The listing builds one solid part. Answer for the finished solid, in the listing's coordinates (mm). Face numbers are marked on the shaded views. Give positions to 0.01 mm unless a question says otherwise; leave off trailing zeros. Loops run counter-clockwise (first coordinate to the right, second up) from the corner with the lowest first, then second, coordinate; pieces in that order, holes last. Notation, with made-up numbers: (0, 18) - (10, 18) arc R20 cw to (10, 37) - close; hole circle Ø8 at (8.25, 32.5). An arc over 180 degrees is marked (long way). Write each question's results on one line, items separated by ' | '.
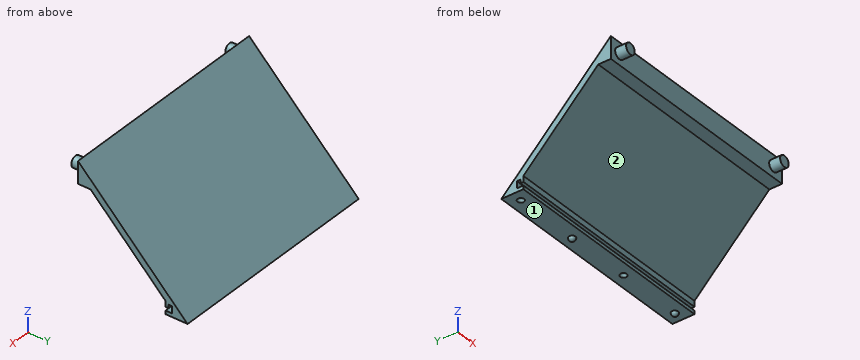
Autodesk Inventor part; units mm, degrees
sketch "Sketch1" plane through (0, 0, 0) normal (1, 0, 0) x (0, 1, 0)
  line L0 (25, 25) -> (-25, 25)
  line L1 (-25, 25) -> (-25, -25)
  line L2 (-25, -25) -> (25, -25)
  line L3 (25, -25) -> (25, 25)
  line L4 (-35, 0) -> (35, 0)
  line L5 (0, 35) -> (0, -35)
  line L6 (-25, 25) -> (25, -25)
  line L7 (-19.2426, 15) -> (14.9373, -19.1799)
  line L8 (-19.2426, 15) -> (-25, 15)
  line L9 (14.9373, -25) -> (14.9373, -19.1799)
  line L10 (14.9373, -21.8) -> (17.9373, -21.8)
  line L11 (17.9373, -21.8) -> (17.9373, -23.4)
  line L12 (17.9373, -23.4) -> (14.9373, -23.4)
  line L13 (14.9373, -23.4) -> (14.9373, -21.8)
  line L14 (17.9373, -21.8) -> (16.3373, -21.8)
  line L15 (16.3373, -21.8) -> (16.3373, -20.2)
  line L16 (16.3373, -20.2) -> (17.9373, -20.2)
  line L17 (17.9373, -20.2) -> (17.9373, -21.8)
  point P0 (0, 0)
  point P1 (25, 0)
  point P2 (0, 25)
  point P3 (20.7574, -25)
  point P4 (-25, 20.7574)
  point P5 (0, 0)
  point P6 (0, 0)
  point P7 (0, -4.2426)
  point P8 (-4.2426, 0)
  dimension "d0" = 50
  dimension "d1" = 50
  dimension "d2" = 3
  dimension "d5" = 10
  dimension "d92" = 3
  dimension "d93" = 1.6
  dimension "d94" = 1.6
  dimension "d95" = 1.6
  dimension "d96" = 1.6
  dimension "d97" = 1.6
extrude "Extrusion1" add sketch "Sketch1" along normal mid plane 100 contours L6 L4 L7 L8 L1 | L5 L7 L4 | L6 L2 L9 L12 L11 L17 L16 L15 L10 L7 L5
sketch "Sketch4" plane through (50, 25, -25) normal (0, 0, -1) x (-1, 0, 0)
  circle A0 centre (5, -5) radius 1.5
  line L0 (0, -10.0627) -> (0, 0)
  line L1 (0, 0) -> (100, 0)
  line L2 (5, -3.5) -> (5, -6.5)
  circle A1 centre (35, -5) radius 1.5
  line L3 (35, -3.5) -> (35, -6.5)
  circle A2 centre (65, -5) radius 1.5
  line L4 (65, -3.5) -> (65, -6.5)
  circle A3 centre (95, -5) radius 1.5
  line L5 (95, -3.5) -> (95, -6.5)
  point P0 (50, -25)
  point P1 (0, -50)
  dimension "d45" = 3
  dimension "d46" = 5
  dimension "d47" = 5
  dimension "d48" = 3
  dimension "d98" = 3
  dimension "d99" = 5
  dimension "d100" = 30
  dimension "d101" = 3
  dimension "d104" = 60
revolve "Revolution2" add sketch "Sketch4" angle 360 about axis through (45, 21.5, -25) along (0, -1, 0) picked at (4.5036, -4.9397) contours L2 A0
revolve "Revolution3" cut sketch "Sketch4" angle 360 about axis through (15, 21.5, -25) along (0, -1, 0) picked at (34.5036, -5.0603) contours L3 A1
revolve "Revolution4" add sketch "Sketch4" angle 360 about axis through (-15, 21.5, -25) along (0, -1, 0) picked at (64.2365, -5.2413) contours L4 A2
revolve "Revolution5" cut sketch "Sketch4" angle 360 about axis through (-45, 21.5, -25) along (0, -1, 0) picked at (94.1238, -4.716) contours L5 A3
sketch "Sketch5" plane through (-50, -25, 15) normal (0, -1, 0) x (1, 0, 0)
  circle A0 centre (5, 5) radius 2.5
  line L0 (0, 0) -> (0, 10)
  line L1 (0, 10) -> (100, 10)
  line L2 (50, 20) -> (50, -50)
  circle A1 centre (95, 5) radius 2.5
  line L3 (0, 5) -> (100, 5)
  line L4 (100, -40) -> (100, 10)
  point P0 (50, -15)
  dimension "d73" = 5
  dimension "d74" = 5
extrude "Extrusion3" add sketch "Sketch5" along normal blind 5 contours L3 A0 | A0 L3 | L3 A1 | A1 L3
properties part number "Roof_Small"
Item 1: Flat-ended cylindrical pins translate along their axes: P1, Ø0.8, axis at x = 24.5, y = 17.5, coming from the -Z side; P2, Ø2.5, axis at x = 12, z = -21, coming from the -Y side; P3, Ø2, axis at x = 29, z = -0.5, coming from the +Y side; P4, Ø12, axis at y = -19, z = -1, coming from the +X side. Find the tip coordinate at first contact, or state that the pin passes through.
Values found:
P1: stops at z = -25 | P2: stops at y = 14.94 | P3: stops at y = 1.5 | P4: passes through
Item 2: Find the intervals of material crossed by line 1 along Z through (x, y) = (-32.5, 16.5); line 2 along Z through (x, y) = (-42, -18); line 3 along Z through (x, y) = (38.5, 17), in increasing order. Write a range as [from, to].
Values found:
line 1: z = [-25, -23.4], [-20.2, -16.5] | line 2: z = [13.76, 18] | line 3: z = [-25, -23.4], [-20.2, -17]
Item 3: A cutting plane is placed at A-A, the plane x = 45. Determine the outline of the cut face in (y, z), plus the area to 3 significant figures.
Values found:
outline: (-30, 17.5) - (-25, 17.5) - (-25, 15) - (-19.24, 15) - (14.94, -19.18) - (14.94, -21.8) - (16.34, -21.8) - (16.34, -20.2) - (17.94, -20.2) - (17.94, -23.4) - (14.94, -23.4) - (14.94, -25) - (18.5, -25) arc R1.5 ccw to (21.5, -25) - (25, -25) - (-25, 25) - (-25, 22.5) - (-30, 22.5) - close | area: 258 mm²
Item 4: A cutting plane is placed at C-C, the plane x = -45. Determine the outline of the cut face in (y, z).
Values found:
outline: (-30, 17.5) - (-25, 17.5) - (-25, 15) - (-19.24, 15) - (14.94, -19.18) - (14.94, -21.8) - (16.34, -21.8) - (16.34, -20.2) - (17.94, -20.2) - (17.94, -23.4) - (14.94, -23.4) - (14.94, -25) - (18.5, -25) arc R1.5 cw to (21.5, -25) - (25, -25) - (-25, 25) - (-25, 22.5) - (-30, 22.5) - close
Item 5: For a pull along X with two mould halves and no side action, classify the marked faces 1 and 2 as released by +X, released by -X, zero draft, split by the parting line, or undercut.
Values found:
face 1: undercut | face 2: zero draft
Item 6: A cutting plane is placed at B-B, the plane z = 20. Determine the outline of the cut face in (x, y), plus the area to 3 significant figures.
Values found:
outline: (-50, -25) - (-47.5, -25) - (-47.5, -30) - (-42.5, -30) - (-42.5, -25) - (42.5, -25) - (42.5, -30) - (47.5, -30) - (47.5, -25) - (50, -25) - (50, -20) - (-50, -20) - close | area: 550 mm²
Item 7: A cutting plane is placed at D-D, the plane y = 11.5. Determine the outline of the cut face in (x, z), plus the area to 3 significant figures.
Values found:
outline: (-50, -15.74) - (50, -15.74) - (50, -11.5) - (-50, -11.5) - close | area: 424 mm²
